Source: CAD feature listing. Evaluate the final solid. Frame: model axes, mm. A direction names the side the tool comes from. Coordinates: 2 decimals unless noted, no trailing zeros. Order: outer loops, then holes, each group sorted by start corner. A loop starts at its lowest first (then second) coordinate and runs counter-clockwise, first axis right, second up.
Autodesk Inventor part; units mm, degrees
ref_plane "YZ Plane" through (0, 0, 0) normal (1, 0, 0) x (0, 1, 0)
ref_plane "XZ Plane" through (0, 0, 0) normal (0, 1, 0) x (-1, 0, 0)
ref_plane "XY Plane" through (0, 0, 0) normal (0, 0, 1) x (1, 0, 0)
sketch "Sketch1" plane through (0, 0, 0) normal (0, 1, 0) x (-1, 0, 0)
  point P0 (0, 0)
sketch "Sketch2" plane through (0, 0, 0) normal (0, 1, 0) x (-1, 0, 0)
  line L0 (5.8709, 8.8623) -> (-86.1291, 8.8623)
  line L1 (-86.1291, 8.8623) -> (-86.1291, 89.8623)
  line L2 (-86.1291, 89.8623) -> (5.8709, 89.8623)
  line L3 (5.8709, 89.8623) -> (5.8709, 8.8623)
  line L4 (1.8709, 85.8623) -> (-82.1291, 85.8623)
  line L5 (-82.1291, 85.8623) -> (-82.1291, 12.8623)
  line L6 (-82.1291, 12.8623) -> (1.8709, 12.8623)
  line L7 (1.8709, 12.8623) -> (1.8709, 85.8623)
  point P0 (0, 0)
  dimension "d0" = 92
  dimension "d1" = 81
  dimension "d4" = 84
  dimension "d5" = 73
extrude "Extrusion1" add sketch "Sketch2" along normal blind 4 contours L0 L1 L2 L3 | L7 L6 L5 L4
sketch "Sketch3" plane through (0, 4, 0) normal (0, 1, 0) x (1, 0, 0)
  line L0 (-5.8709, -89.8623) -> (86.1291, -89.8623)
  line L1 (-1.8709, -89.8623) -> (2.1291, -89.8623) construction
  line L2 (-1.8709, -85.8623) -> (82.1291, -85.8623)
  line L3 (82.1291, -85.8623) -> (82.1291, -12.8623)
  line L4 (82.1291, -12.8623) -> (-1.8709, -12.8623)
  line L5 (-1.8709, -12.8623) -> (-1.8709, -85.8623)
  line L6 (86.1291, -89.8623) -> (86.1291, -8.8623)
  line L7 (-5.8709, -89.8623) -> (86.1291, -89.8623)
  line L8 (86.1291, -89.8623) -> (86.1291, -8.8623)
  line L9 (86.1291, -8.8623) -> (-5.8709, -8.8623)
  line L10 (-5.8709, -8.8623) -> (-5.8709, -89.8623)
  point P0 (0, 0)
  dimension "d9" = 4
  dimension "d11" = 84
  dimension "d12" = 73
extrude "Extrusion2" add sketch "Sketch3" along normal blind 216
fillet "Fillet1" radius 2 8 edges at (86.1291, 110, 89.8623) (86.1291, 110, 8.8623) (-5.8709, 110, 8.8623) (-5.8709, 110, 89.8623) (40.1291, 0, 89.8623) (86.1291, 0, 49.3623) (40.1291, 0, 8.8623) (-5.8709, 0, 49.3623)
properties part number "Battery Box Top_3DPrint"
1. Contact query for flat-ended pins moving along their axis: P1, Ø6, axis at x = 11, z = 51.5, coming from the -Y side; P2, Ø5, axis at x = 11.5, z = 44, coming from the +Y side. Output: stop coordinate, or through.
2. Section query C-C, the plane x = 19. Output: boundary loops of the cut face in (y, z), plus the area to 3 significant figures.
3. Access query for faces 1 (the flat face through (41, 109, 8.862)), 2 (the flat face through (41, 4, 50)). Directions: +Z, -Z, +X, -X, +Y, -Y. A direction counts if a zero-diameter tool reaches every point of the face in a straight line with its end or side. Return the directions, or none.
4. Section query B-B, the plane z = 58.5. Output: boundary loops of the cut face in (x, y).
5. Section query A-A, the plane y = 153. Output: boundary loops of the cut face in (x, z), plus the area to 3 significant figures.
6. Material intervals for line 1 along Z through (x, y) = (2, 81); line 2 along X through (y, z) = (194.5, 41); line 3 along Y through (x, z) = (10, 53), sorted ascending.
Answer key:
1. P1: stops at y = 0
1. P2: stops at y = 4
2. outline: (0, 10.86) arc R2 ccw to (2, 8.86) - (220, 8.86) - (220, 12.86) - (4, 12.86) - (4, 85.86) - (220, 85.86) - (220, 89.86) - (2, 89.86) arc R2 ccw to (0, 87.86) - close
2. area: 2,050 mm2
3. face 1: -Z, +X, -X, +Y, -Y
3. face 2: +Y
4. outline: (-5.87, 2) arc R2 ccw to (-3.87, 0) - (84.13, 0) arc R2 ccw to (86.13, 2) - (86.13, 220) - (82.13, 220) - (82.13, 4) - (-1.87, 4) - (-1.87, 220) - (-5.87, 220) - close
5. outline: (-5.87, 10.86) arc R2 ccw to (-3.87, 8.86) - (84.13, 8.86) arc R2 ccw to (86.13, 10.86) - (86.13, 87.86) arc R2 ccw to (84.13, 89.86) - (-3.87, 89.86) arc R2 ccw to (-5.87, 87.86) - close; hole (-1.87, 12.86) - (82.13, 12.86) - (82.13, 85.86) - (-1.87, 85.86) - close
5. area: 1,320 mm2
6. line 1: z = 8.86 to 12.86, 85.86 to 89.86
6. line 2: x = -5.87 to -1.87, 82.13 to 86.13
6. line 3: y = 0 to 4
